from build123d import *
from build123d.topology import SkipClean

# Parameters (mm, degrees)
SKETCH1_W             = 48
SKETCH1_H             = 53
BOSS_EXTRUDE1_DEPTH   = 10
SKETCH2_W             = 48
SKETCH2_H             = 5.616325
BOSS_EXTRUDE2_DEPTH   = 33.1917878
SKETCH4_W             = 4
SKETCH4_H             = 10
BOSS_EXTRUDE4_DEPTH   = 40
SKETCH5_W             = 48
SKETCH5_H             = 10.8609375
BOSS_EXTRUDE5_DEPTH   = 23.1917878
SKETCH6_W             = 48
SKETCH6_H             = 5
BOSS_EXTRUDE6_DEPTH   = 42.3
SKETCH7_W             = 12.8082122
SKETCH7_H             = 16.4772625
BOSS_EXTRUDE7_DEPTH   = 48
CUT_EXTRUDE1_REACH    = 84.426
SKETCH8_R             = 11.5
SKETCH8_R_2           = 2
FILLET1_R             = 10
FILLET2_R             = 4
SKETCH9_W             = 5
SKETCH9_H             = 16.4772625
BOSS_EXTRUDE9_DEPTH   = 48
CUT_EXTRUDE2_DEPTH    = 88.252507127
SKETCH11_W            = 51
SKETCH11_H            = 16.4772625
BOSS_EXTRUDE10_DEPTH  = 49.45
BOSS_EXTRUDE11_DEPTH  = 46
SKETCH16_W            = 47.95
SKETCH16_H            = 51
BOSS_EXTRUDE14_DEPTH  = 2.55
SKETCH14_W            = 5
SKETCH14_H            = 42.3
BOSS_EXTRUDE13_DEPTH  = 1.5
SKETCH17_W            = 51
SKETCH17_H            = 19.0272625
BOSS_EXTRUDE15_DEPTH  = 9
BOSS_EXTRUDE16_DEPTH  = 25
SKETCH19_R            = 1.9304
CUT_EXTRUDE3_DEPTH    = 125.404890183
MIRROR2_START         = 33.1917878
MIRROR2_DEPTH         = 51
MIRROR2_START_2       = 76.1917878
MIRROR2_2_OUTLINE_W   = 47.95
MIRROR2_2_OUTLINE_H   = 25
MIRROR2_2_OUTLINE_R   = 1.9304
MIRROR2_2_DEPTH       = 8
MIRROR2_3_OUTLINE_W   = 45
MIRROR2_3_OUTLINE_H   = 42.3
MIRROR2_3_OUTLINE_R   = 2
MIRROR2_3_OUTLINE_R_2 = 11.5
MIRROR2_3_DEPTH       = 5
SKETCH20_W            = 103.287975037
SKETCH20_H            = 97.84889924
CUT_EXTRUDE4_DEPTH    = 144.929961559
SKETCH21_W            = 49.5
SKETCH21_H            = 42.3
CUT_EXTRUDE5_DEPTH    = 128.391431036
SKETCH24_R            = 7.5
BOSS_EXTRUDE18_DEPTH  = 45
BOSS_EXTRUDE19_DEPTH  = 29
SKETCH26_R            = 3.937
CUT_EXTRUDE6_DEPTH    = 135.023808387


# Read off the part's stored shape, not the designer's step: Mirror2
with BuildPart() as part:
    # Sketch1 → Boss-Extrude1 (new body)
    with BuildSketch(Plane.XY):
        with Locations((24, 26.5)):
            Rectangle(SKETCH1_W, SKETCH1_H)
    extrude(amount=BOSS_EXTRUDE1_DEPTH)

    # Sketch2 → Boss-Extrude2 (add)
    with BuildSketch(Plane(origin=(0, 0, 0), x_dir=(-1, 0, 0), z_dir=(0, 0, -1))):
        with Locations((-24, -2.8081625)):
            Rectangle(SKETCH2_W, SKETCH2_H)
    extrude(amount=-BOSS_EXTRUDE2_DEPTH)

    # Sketch4 → Boss-Extrude4 (add)
    with BuildSketch(Plane.XY.offset(10)):
        with Locations((2, 48)):
            Rectangle(SKETCH4_W, SKETCH4_H)
        with Locations((46, 48)):
            Rectangle(SKETCH4_W, SKETCH4_H)
    extrude(amount=BOSS_EXTRUDE4_DEPTH)

    # Sketch5 → Boss-Extrude5 (add)
    with BuildSketch(Plane.XY.offset(10)):
        with Locations((24, 5.43046875)):
            Rectangle(SKETCH5_W, SKETCH5_H)
    extrude(amount=BOSS_EXTRUDE5_DEPTH)

    # Sketch6 → Boss-Extrude6 (add)
    with BuildSketch(Plane.XZ.offset(5.616325)):
        with Locations((24, 30.6917878)):
            Rectangle(SKETCH6_W, SKETCH6_H)
    extrude(amount=BOSS_EXTRUDE6_DEPTH)

    # Sketch7 → Boss-Extrude7 (add)
    with BuildSketch(Plane.ZY):
        with Locations((-6.4041061, 2.62230625)):
            Rectangle(SKETCH7_W, SKETCH7_H)
    extrude(amount=-BOSS_EXTRUDE7_DEPTH)

    # Sketch8 → Cut-Extrude1 (cut, up to next)
    with BuildSketch(Plane(origin=(0, 0, 28.1917878), x_dir=(-1, 0, 0), z_dir=(0, 0, -1)), mode=Mode.PRIVATE) as cut_extrude1_sk1:
        with Locations((-24, -26.616325)):
            Circle(SKETCH8_R)
    cut_extrude1_tool1 = extrude(cut_extrude1_sk1.sketch, amount=-CUT_EXTRUDE1_REACH, mode=Mode.PRIVATE) & part.part
    # Sketch8 → Cut-Extrude1 (cut, up to next)
    with BuildSketch(Plane(origin=(0, 0, 28.1917878), x_dir=(-1, 0, 0), z_dir=(0, 0, -1)), mode=Mode.PRIVATE) as cut_extrude1_sk2:
        with Locations((-39.5, -11.116325)):
            Circle(SKETCH8_R_2)
    cut_extrude1_tool2 = extrude(cut_extrude1_sk2.sketch, amount=-CUT_EXTRUDE1_REACH, mode=Mode.PRIVATE) & part.part
    # Sketch8 → Cut-Extrude1 (cut, up to next)
    with BuildSketch(Plane(origin=(0, 0, 28.1917878), x_dir=(-1, 0, 0), z_dir=(0, 0, -1)), mode=Mode.PRIVATE) as cut_extrude1_sk3:
        with Locations((-39.5, -42.116325)):
            Circle(SKETCH8_R_2)
    cut_extrude1_tool3 = extrude(cut_extrude1_sk3.sketch, amount=-CUT_EXTRUDE1_REACH, mode=Mode.PRIVATE) & part.part
    # Sketch8 → Cut-Extrude1 (cut, up to next)
    with BuildSketch(Plane(origin=(0, 0, 28.1917878), x_dir=(-1, 0, 0), z_dir=(0, 0, -1)), mode=Mode.PRIVATE) as cut_extrude1_sk4:
        with Locations((-8.5, -11.116325)):
            Circle(SKETCH8_R_2)
    cut_extrude1_tool4 = extrude(cut_extrude1_sk4.sketch, amount=-CUT_EXTRUDE1_REACH, mode=Mode.PRIVATE) & part.part
    # Sketch8 → Cut-Extrude1 (cut, up to next)
    with BuildSketch(Plane(origin=(0, 0, 28.1917878), x_dir=(-1, 0, 0), z_dir=(0, 0, -1)), mode=Mode.PRIVATE) as cut_extrude1_sk5:
        with Locations((-8.5, -42.116325)):
            Circle(SKETCH8_R_2)
    cut_extrude1_tool5 = extrude(cut_extrude1_sk5.sketch, amount=-CUT_EXTRUDE1_REACH, mode=Mode.PRIVATE) & part.part
    add(cut_extrude1_tool1.solids().sort_by_distance((24, -26.616325, 28.191788))[0], mode=Mode.SUBTRACT)
    add(cut_extrude1_tool2.solids().sort_by_distance((39.5, -11.116325, 28.191788))[0], mode=Mode.SUBTRACT)
    add(cut_extrude1_tool3.solids().sort_by_distance((39.5, -42.116325, 28.191788))[0], mode=Mode.SUBTRACT)
    add(cut_extrude1_tool4.solids().sort_by_distance((8.5, -11.116325, 28.191788))[0], mode=Mode.SUBTRACT)
    add(cut_extrude1_tool5.solids().sort_by_distance((8.5, -42.116325, 28.191788))[0], mode=Mode.SUBTRACT)

    # Fillet1
    fillet1_edges = [part.edges().sort_by_distance(p)[0] for p in [
        (24, 10.8609375, 0),
    ]]
    fillet(fillet1_edges, radius=FILLET1_R)

    # Fillet2
    fillet2_edges = [part.edges().sort_by_distance(p)[0] for p in [
        (2, 43, 10),
        (46, 43, 10),
    ]]
    fillet(fillet2_edges, radius=FILLET2_R)

    # Sketch9 → Boss-Extrude9 (add)
    with BuildSketch(Plane(origin=(48, 0, 0), x_dir=(0, 0, -1), z_dir=(1, 0, 0))):
        with Locations((15.3082122, 2.62230625)):
            Rectangle(SKETCH9_W, SKETCH9_H)
    extrude(amount=-BOSS_EXTRUDE9_DEPTH)

    # Sketch10 → Cut-Extrude2 (cut, through all)
    with BuildSketch(Plane(origin=(48, 0, 0), x_dir=(0, 0, -1), z_dir=(1, 0, 0))):
        Polygon((17.8082122, 10.8609375), (-33.1917878, 10.8609375), (-76.887145623, 43.902095521), (-50.794096938, 74.436514195), (27.207463492, 71.105486703), align=None)
    extrude(amount=-CUT_EXTRUDE2_DEPTH, mode=Mode.SUBTRACT)

    # Sketch11 → Boss-Extrude10 (add)
    with BuildSketch(Plane(origin=(48, 0, 0), x_dir=(0, 0, -1), z_dir=(1, 0, 0))):
        with Locations((-7.6917878, 2.62230625)):
            Rectangle(SKETCH11_W, SKETCH11_H)
    extrude(amount=BOSS_EXTRUDE10_DEPTH)

    # Sketch12 → Boss-Extrude11 (add)
    with BuildSketch(Plane(origin=(0, 0, 28.1917878), x_dir=(-1, 0, 0), z_dir=(0, 0, -1))):
        Polygon((-48, -47.916325), (-45, -47.916325), (-45, -5.616325), (-49.5, -5.616325), (-49.5, -47.916325), align=None)
    extrude(amount=BOSS_EXTRUDE11_DEPTH)

    # Sketch16 → Boss-Extrude14 (add)
    with BuildSketch(Plane.XZ.offset(5.616325)):
        with Locations((73.475, 7.6917878)):
            Rectangle(SKETCH16_W, SKETCH16_H)
    extrude(amount=BOSS_EXTRUDE14_DEPTH)

    # Sketch14 → Boss-Extrude13 (add)
    with BuildSketch(Plane(origin=(49.5, 0, 0), x_dir=(0, 0, -1), z_dir=(1, 0, 0))):
        with Locations((-30.6917878, -26.766325)):
            Rectangle(SKETCH14_W, SKETCH14_H)
    extrude(amount=-BOSS_EXTRUDE13_DEPTH)

    # Sketch17 → Boss-Extrude15 (add)
    with BuildSketch(Plane(origin=(97.45, 0, 0), x_dir=(0, 0, -1), z_dir=(1, 0, 0))):
        with Locations((-7.6917878, 1.34730625)):
            Rectangle(SKETCH17_W, SKETCH17_H)
    extrude(amount=BOSS_EXTRUDE15_DEPTH)

    # Sketch18 → Boss-Extrude16 (add)
    with BuildSketch(Plane.XZ.offset(8.166325)):
        Polygon((49.5, -17.8082122), (106.45, -17.8082122), (106.45, -9.8082122), (106.45, 33.1917878), (97.45, 33.1917878), (97.45, -9.8082122), (49.5, -9.8082122), align=None)
    extrude(amount=BOSS_EXTRUDE16_DEPTH)

    # Sketch19 → Cut-Extrude3 (cut, through all)
    with BuildSketch(Plane.XY.offset(-9.8082122)):
        with Locations((58.475, -26.166325)):
            Circle(SKETCH19_R)
        with Locations((88.475, -26.166325)):
            Circle(SKETCH19_R)
    extrude(amount=-CUT_EXTRUDE3_DEPTH, mode=Mode.SUBTRACT)

    # Mirror2 outline → Mirror2 (add)
    with BuildSketch(Plane.XY.offset(MIRROR2_START)):
        Polygon((49.5, -47.916325), (49.5, -8.166325), (97.45, -8.166325), (97.45, -33.166325), (106.45, -33.166325), (106.45, 10.8609375), (0, 10.8609375), (0, -5.616325), (45, -5.616325), (45, -47.916325), align=None)
    extrude(amount=MIRROR2_DEPTH)

    # Mirror2 2 outline → Mirror2 2 (add)
    with BuildSketch(Plane.XY.offset(MIRROR2_START_2)):
        with Locations((73.475, -20.666325)):
            Rectangle(MIRROR2_2_OUTLINE_W, MIRROR2_2_OUTLINE_H)
        with Locations((58.475, -26.166325)):
            Circle(MIRROR2_2_OUTLINE_R, mode=Mode.SUBTRACT)
        with Locations((88.475, -26.166325)):
            Circle(MIRROR2_2_OUTLINE_R, mode=Mode.SUBTRACT)
    extrude(amount=MIRROR2_2_DEPTH)

    # Mirror2 3 outline → Mirror2 3 (add)
    with SkipClean():  # the faces are left unmerged after this step: merging them gives an invalid solid
        with BuildSketch(Plane.XY.offset(MIRROR2_START)):
            with Locations((22.5, -26.766325)):
                Rectangle(MIRROR2_3_OUTLINE_W, MIRROR2_3_OUTLINE_H)
            with Locations((8.5, -42.116325)):
                Circle(MIRROR2_3_OUTLINE_R, mode=Mode.SUBTRACT)
            with Locations((39.5, -42.116325)):
                Circle(MIRROR2_3_OUTLINE_R, mode=Mode.SUBTRACT)
            with Locations((24, -26.616325)):
                Circle(MIRROR2_3_OUTLINE_R_2, mode=Mode.SUBTRACT)
            with Locations((8.5, -11.116325)):
                Circle(MIRROR2_3_OUTLINE_R, mode=Mode.SUBTRACT)
            with Locations((39.5, -11.116325)):
                Circle(MIRROR2_3_OUTLINE_R, mode=Mode.SUBTRACT)
        extrude(amount=MIRROR2_3_DEPTH)

    # Sketch20 → Cut-Extrude4 (cut, through all)
    with BuildSketch(Plane.ZY):
        with Locations((-18.452199719, -38.06351212)):
            Rectangle(SKETCH20_W, SKETCH20_H)
    extrude(amount=-CUT_EXTRUDE4_DEPTH, mode=Mode.SUBTRACT)

    # Sketch21 → Cut-Extrude5 (cut, through all)
    with BuildSketch(Plane.XY.offset(84.1917878)):
        with Locations((24.75, -26.766325)):
            Rectangle(SKETCH21_W, SKETCH21_H)
    extrude(amount=-CUT_EXTRUDE5_DEPTH, mode=Mode.SUBTRACT)



with BuildPart() as body_2:
    # Sketch24 → Boss-Extrude18 (new body)
    with BuildSketch(Plane.XY.offset(55.1917878)):
        with Locations((24, -29.616325)):
            Circle(SKETCH24_R)
    extrude(amount=-BOSS_EXTRUDE18_DEPTH)


with BuildPart() as part_1:
    add(part.part)

    add(body_2.part)  # Boss-Extrude19 merges body 2
    # Sketch25 → Boss-Extrude19 (add)
    with BuildSketch(Plane.XY.offset(55.1917878)):
        with BuildLine():
            Line((16.5, -29.616325), (12.268152463, -5.616325))
            Line((12.268152463, -5.616325), (35.731847537, -5.616325))
            Line((35.731847537, -5.616325), (31.5, -29.616325))
            ThreePointArc((31.5, -29.616325), (24, -37.116325), (16.5, -29.616325))
        make_face()
    extrude(amount=BOSS_EXTRUDE19_DEPTH)

    # Sketch26 → Cut-Extrude6 (cut, through all)
    with BuildSketch(Plane.ZY.offset(-97.45)):
        with Locations((59.1917878, -16.166325)):
            Circle(SKETCH26_R)
    extrude(amount=-CUT_EXTRUDE6_DEPTH, mode=Mode.SUBTRACT)


solid = part_1.part
Here's how the part is built. I have some questions about the finished solid (model axes, mm). A direction names the side the tool comes from. Round coordinates to 2 decimals unless told otherwise and drop trailing zeros. Write each loop counter-clockwise with the first axis right and the second up, starting at its lowest first coordinate (ties: lowest second). Pieces come first, ordered by that corner, then holes. Notation, with made-up numbers: (84, 59.5) -> (109, 59.5) arc R27 ccw to (109, 78.5) -> close; hole circle Ø2 at (-0.75, -3.5). An arc over 180 degrees is marked (long way). One line per item, written item: value.
1) If I drill on line 1 (Z direction, x = 99, y = -11); line 2 (Y direction, x = 63.5, z = 77); line 3 (Y direction, x = 85, z = 37), over which ranges is the centre line in solid material (lowest first)? Write a range as [from, to].
Filled sheet:
line 1: z = [33.19, 84.19]
line 2: y = [-33.17, 10.86]
line 3: y = [-8.17, 10.86]
2) Suppose I cut it at C-C on x = 24. List the corners of the cut face in (y, z) for me, plus the area to 3 significant figures.
Filled sheet:
outline: (-37.12, 10.19) -> (-22.12, 10.19) -> (-22.12, 55.19) -> (-5.62, 55.19) -> (-5.62, 33.19) -> (10.86, 33.19) -> (10.86, 84.19) -> (-37.12, 84.19) -> close
area: 2,430 mm2
3) We'd pull the mould along X, two halves only. Please class faces 4 (the face through (106.45, -11, 58)), 5 (the face through (0, 3, 58)), 6 (the face through (24, -5.616, 53)), 7 (the face through (101.887, -18.562, 56.068)): released by +X, released by -X, zero draft, split by the parting line, or undercut.
Filled sheet:
face 4: released by +X
face 5: released by -X
face 6: undercut
face 7: zero draft
4) Suppose I cut it at D-D on y = -10.5. List the corners of the cut face in (x, z) for me, plus the area to 3 significant figures.
Filled sheet:
outline: (13.13, 55.19) -> (34.87, 55.19) -> (34.87, 84.19) -> (13.13, 84.19) -> close; (49.5, 76.19) -> (97.45, 76.19) -> (97.45, 33.19) -> (106.45, 33.19) -> (106.45, 84.19) -> (49.5, 84.19) -> close
area: 1,470 mm2
5) For faces 1 (the face through (97.45, -20, 54)), 2 (the face through (23.024, -37.053, 38.452)), 3 (the face through (86, -33.166, 77)), which set-ups out of +Z, -Z, +X, -X, +Y, -Y let a thin tool reach every point of the face, with its end or its side?
Filled sheet:
face 1: -Z, -Y
face 2: -Z
face 3: +Z, -Z, +X, -Y
6) Suppose I cut it at B-B on y = -18. List the corners of the cut face in (x, z) for me, plus the area to 3 significant figures.
Filled sheet:
outline: (14.45, 55.19) -> (33.55, 55.19) -> (33.55, 84.19) -> (14.45, 84.19) -> close; (49.5, 76.19) -> (97.45, 76.19) -> (97.45, 62.68) -> (106.45, 62.68) -> (106.45, 84.19) -> (49.5, 84.19) -> close; (97.45, 33.19) -> (106.45, 33.19) -> (106.45, 55.71) -> (97.45, 55.71) -> close
area: 1,330 mm2
7) I'm going to push flat-ended pins straight in: pin 1 Ø3 at (y, z) = (-25.5, 53) entering from -X; pin 2 Ø10 at (y, z) = (-20.5, 63) entering from -X; pin 3 Ø7 at (x, y) = (27, -18.5) entering from -Z. Where does each tip first touch, or does it pass through?
Filled sheet:
pin 1: stops at x = 16.97
pin 2: stops at x = 14.01
pin 3: stops at z = 55.19
8) Suppose I cut it at A-A on z = 51.5. List the corners of the cut face in (x, y) for me.
Filled sheet:
outline: (0, -5.62) -> (49.5, -5.62) -> (49.5, -8.17) -> (97.45, -8.17) -> (97.45, -33.17) -> (106.45, -33.17) -> (106.45, 10.86) -> (0, 10.86) -> close; circle Ø15 at (24, -29.62)
